Autodesk Inventor part; units mm, degrees
ref_plane "YZ Plane" through (0, 0, 0) normal (1, 0, 0) x (0, 1, 0)
ref_plane "XZ Plane" through (0, 0, 0) normal (0, 1, 0) x (-1, 0, 0)
ref_plane "XY Plane" through (0, 0, 0) normal (0, 0, 1) x (1, 0, 0)
sketch "Sketch1" plane through (0, 0, 0) normal (0, 0, 1) x (1, 0, 0)
  line L0 (-3.6662, 6.35) -> (3.6662, 6.35)
  line L1 (3.6662, 6.35) -> (7.3323, 0)
  line L2 (7.3323, 0) -> (3.6662, -6.35)
  line L3 (3.6662, -6.35) -> (-3.6662, -6.35)
  line L4 (-3.6662, -6.35) -> (-7.3323, 0)
  line L5 (-7.3323, 0) -> (-3.6662, 6.35)
  point P0 (0, 0)
  point P1 (0, 0)
  dimension "d0" = 12.7
extrude "Extrusion1" add sketch "Sketch1" along normal mid plane 38.1
sketch "Sketch2" plane through (0, 0, 19.05) normal (0, 0, 1) x (1, 0, 0)
  point P0 (0, 0)
  point P1 (0, 0)
hole "Hole1" at (0, 0, 19.05) direction (0, 0, -1) diameter 4.9784 end through all
properties part number "Hex Standoff 14-20 x1500" material "Aluminum 6061"
Build history of the part. All positions in model axes, mm. Give positions to 0.01 mm unless a question says otherwise; leave off trailing zeros. Loops run counter-clockwise (first coordinate to the right, second up) from the corner with the lowest first, then second, coordinate; pieces in that order, holes last. Notation, with made-up numbers: (43.25, 53) -> (89.25, 53) arc R23 ccw to (89.25, 75) -> close; hole circle Ø10 at (72.25, 34.25). An arc over 180 degrees is marked (long way). One line per question, with ' | ' between items.
Q1. Cut at D-D, the plane x = 5.25. Write the cut outline in (y, z), plus the area to 3 significant figures.
Filled sheet:
outline: (-3.61, -19.05) -> (3.61, -19.05) -> (3.61, 19.05) -> (-3.61, 19.05) -> close | area: 275 mm²
Q2. Pull direction Z, two halves, no side cores. Call faces 1 (the flat face through (3, 0, -19.05)), 2 (the flat face through (3, 0, 19.05)), 3 (the flat face through (5.525, -3.131, -0.267)): pulls with the +Z half, pulls with the -Z half, needs draft (parallel to the pull), parting line crosses it, or undercut.
Filled sheet:
face 1: pulls with the -Z half | face 2: pulls with the +Z half | face 3: needs draft
Q3. Drop flat-ended pins along their axis: pin 1 (3 mm diameter, centred on y = 1, z = 12.5, fed in from -X); pin 2 (1 mm diameter, centred on y = 4, z = 14.5, fed in from +X); pin 3 (4.5 mm diameter, centred on x = 0, y = 0, fed in from -Z). Give the stop position or say it passes through.
Filled sheet:
pin 1: stops at x = -7.33 | pin 2: stops at x = 5.31 | pin 3: passes through
Q4. Cut at C-C, the plane y = -1. Write the cut outline in (x, z), plus the area to 3 significant figures.
Filled sheet:
outline: (-6.75, -19.05) -> (-2.28, -19.05) -> (-2.28, 19.05) -> (-6.75, 19.05) -> close; (2.28, -19.05) -> (6.75, -19.05) -> (6.75, 19.05) -> (2.28, 19.05) -> close | area: 341 mm²
Q5. Cut at A-A, the plane x = 0. Write the cut outline in (y, z), plus the area to 3 significant figures.
Filled sheet:
outline: (-6.35, -19.05) -> (-2.49, -19.05) -> (-2.49, 19.05) -> (-6.35, 19.05) -> close; (2.49, -19.05) -> (6.35, -19.05) -> (6.35, 19.05) -> (2.49, 19.05) -> close | area: 294 mm²
Q6. Cut at B-B, the plane z = -15. Write the cut outline in (x, y).
Filled sheet:
outline: (-7.33, 0) -> (-3.67, -6.35) -> (3.67, -6.35) -> (7.33, 0) -> (3.67, 6.35) -> (-3.67, 6.35) -> close; hole circle Ø4.98 at (0, 0)
Q7. Drill centre lines: line 1 along X through (y, z) = (0, 7); line 2 along Y through (x, z) = (0, -10); line 3 along Y through (x, z) = (1.75, 13). Where is each one in solid material? Low to high. Write a range as [from, to].
Filled sheet:
line 1: x = [-7.33, -2.49], [2.49, 7.33] | line 2: y = [-6.35, -2.49], [2.49, 6.35] | line 3: y = [-6.35, -1.77], [1.77, 6.35]
